Autodesk Inventor part; units mm, degrees
ref_plane "YZ Plane" through (0, 0, 0) normal (1, 0, 0) x (0, 1, 0)
ref_plane "XZ Plane" through (0, 0, 0) normal (0, 1, 0) x (-1, 0, 0)
ref_plane "XY Plane" through (0, 0, 0) normal (0, 0, 1) x (1, 0, 0)
sketch "Sketch1" plane through (0, 0, 0) normal (0, 0, 1) x (1, 0, 0)
  line L0 (-20, -20) -> (20, -20)
  line L1 (20, -20) -> (20, 20)
  line L2 (20, 20) -> (-20, 20)
  line L3 (-20, 20) -> (-20, -20)
  line L4 (-20, -20) -> (20, 20) construction
  line L5 (20, -20) -> (-20, 20) construction
  line L6 (-22.5, 22.5) -> (22.5, 22.5)
  line L7 (22.5, 22.5) -> (22.5, -20)
  line L8 (22.5, -20) -> (-22.5, -20)
  line L9 (-22.5, -20) -> (-22.5, 22.5)
  line L10 (-33.9631, 22.5) -> (42.8206, 22.5) construction
  line L11 (-22.5, 22.5) -> (4.744, 22.5) construction
  line L12 (4.744, 22.5) -> (22.5, 22.5) construction
  line L13 (22.5, 22.5) -> (22.5, 26.484) construction
  line L14 (22.5, 26.484) -> (4.744, 26.484) construction
  line L15 (4.744, 26.484) -> (4.744, 22.5) construction
  arc A0 (4.744, 22.5) -> (22.5, 26.484) centre (4.7442, 64.059) ccw
  line L16 (22.5, 26.484) -> (22.5, 22.5)
  line L17 (22.5, 22.5) -> (4.744, 22.5)
  point P0 (0, 0)
  dimension "d0" = 40
  dimension "d1" = 40
  dimension "d2" = 2.5
  dimension "d3" = 42.5
  dimension "d4" = 2.5
  dimension "d5" = 2.5
  dimension "d6" = 27.244
  dimension "d7" = 3.984
  dimension "d8" = 41.559
extrude "Extrusion1" add sketch "Sketch1" along normal blind 112.1 contours L8 L9 L6 L7 L1 L2 L3 | L6 A0 L16
sketch "Sketch2" plane through (-20, 20, 0) normal (0, -1, 0) x (1, 0, 0)
  line L0 (0, 0) -> (0, 112.1) construction
  line L1 (40, 112.1) -> (40, 0) construction
  line L2 (0, 112.1) -> (40, 112.1) construction
  line L3 (40, 112.1) -> (40, 0) construction
  line L4 (40, 0) -> (0, 0) construction
  line L5 (0, 0) -> (0, 112.1) construction
  line L6 (20, 112.1) -> (20, 0) construction
  line L7 (24.744, 0) -> (24.744, 112.1) construction
  line L8 (42.5, 0) -> (40, 0) construction
  line L9 (0, 112.1) -> (40, 0) construction
  line L10 (0, 0) -> (40, 112.1) construction
  line L11 (40, 56.05) -> (0, 112.1) construction
  line L12 (0, 56.05) -> (40, 112.1) construction
  line L13 (0, 56.05) -> (40, 0) construction
  line L14 (40, 56.05) -> (0, 0) construction
  point P0 (20, 28.025)
  point P1 (20, 84.075)
hole "Hole1" at (0, 20, 28.025) at (0, 20, 84.075) direction (0, 1, 0) diameter 5 depth 8 tip angle 118
fillet "Fillet1" radius 4 2 edges at (20, 20, 56.05) (-20, 20, 56.05)
fillet "Fillet2" radius 2 2 edges at (-22.5, -20, 56.05) (22.5, -20, 56.05)
equation "\"d4\" = d2"
equation "\"d5\" = d4"
properties part number "display_holder"
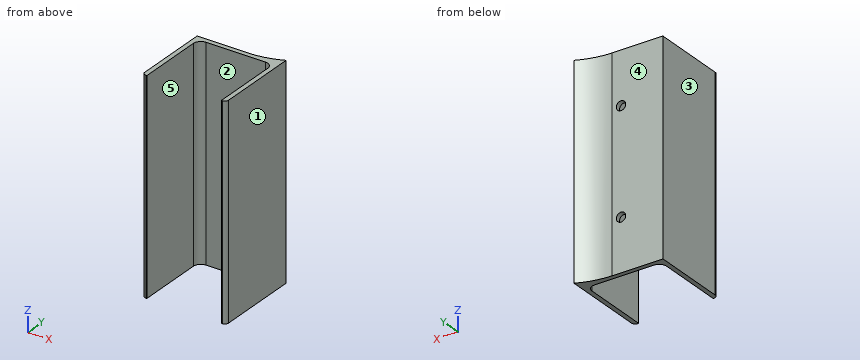
Can you work these out from the model? Positions are in its coordinate system, mm. Face numbers are marked on the shaded views. A direction names the side the tool comes from. Round coordinates to 2 decimals unless told otherwise and drop trailing zeros. Write each loop counter-clockwise with the first axis right and the second up, starting at its lowest first coordinate (ties: lowest second). Pieces come first, ordered by that corner, then holes. Notation, with made-up numbers: (26, -6) -> (56, -6) arc R14 ccw to (56, 12) -> close; hole circle Ø3 at (84, 72). An arc over 180 degrees is marked (long way). One line per question, with ' | ' between items. Start each with the question number.
1) If we mould it in two halves opening along X, with no side actions, what happens to the marked faces 1, 2 and 3? For each: released by +X, released by -X, zero draft, split by the parting line, or undercut.
2) I need wall thicknesses on line 1 (Z direction, x = 0, y = 21.3) (3 decimals); line 2 (X direction, y = -10, z = 22); line 3 (Y direction, x = 4, z = 80). Which ranges of each line are inside material? Lowest first, please. Write a range as [from, to].
3) On a 3-axis mill with a long thin cutter (end or side, diameter ignored), from which of +Z, -Z, +X, -X, +Y, -Y can I reach the whole of each face in a straight line? I mean the marked faces 4 and 5. Say none if no direction works.
4) Suppose I cut it at D-D on x = -9.5. Write out the boundary of the cut face in (y, z), then the cut area to 3 significant figures.
5) Suppose I cut it at B-B on y = 5.5. Write out the boundary of the cut face in (x, z).
6) Suppose I cut it at A-A on x = 0. Write out the boundary of the cut face in (y, z) (3 decimals).
7) Suppose I cut it at C-C on z = 39.5. Write out the boundary of the cut face in (x, y), then the cut area to 3 significant figures.
8) I'm going to push flat-ended pins straight in: P1, Ø5, axis at x = 12.5, z = 83, coming from the +Y side; P2, Ø3, axis at x = 8, z = 26, coming from the -Y side; P3, Ø22, axis at x = -2.5, z = 79, coming from the +Y side. Where does each tip first touch, or does it pass through?
Return value:
1) face 1: released by +X | face 2: undercut | face 3: released by -X
2) line 1: z = [0, 25.525], [30.525, 81.575], [86.575, 112.1] | line 2: x = [-22.5, -20], [20, 22.5] | line 3: y = [20, 22.5]
3) face 4: +Z, -Z, -X, +Y | face 5: +Z, -Z, -Y
4) outline: (20, 0) -> (22.5, 0) -> (22.5, 112.1) -> (20, 112.1) -> close | area: 280 mm2
5) outline: (-22.5, 0) -> (-20, 0) -> (-20, 112.1) -> (-22.5, 112.1) -> close; (20, 0) -> (22.5, 0) -> (22.5, 112.1) -> (20, 112.1) -> close
6) outline: (20, 0) -> (22.5, 0) -> (22.5, 25.525) -> (20, 25.525) -> close; (20, 30.525) -> (22.5, 30.525) -> (22.5, 81.575) -> (20, 81.575) -> close; (20, 86.575) -> (22.5, 86.575) -> (22.5, 112.1) -> (20, 112.1) -> close
7) outline: (-22.5, -18) arc R2 ccw to (-20.5, -20) -> (-20, -20) -> (-20, 16) arc R4 cw to (-16, 20) -> (16, 20) arc R4 cw to (20, 16) -> (20, -20) -> (20.5, -20) arc R2 ccw to (22.5, -18) -> (22.5, 26.48) arc R41.56 cw to (4.74, 22.5) -> (-22.5, 22.5) -> close | area: 341 mm2
8) P1: stops at y = 23.79 | P2: stops at y = 20 | P3: stops at y = 22.67
